The model under review builds one solid part; all positions refer to its coordinate system, in mm. Face numbers are marked on the shaded views. A direction names the side the tool comes from. Coordinates: 2 decimals unless noted, no trailing zeros. Write each loop counter-clockwise with the first axis right and the second up, starting at its lowest first coordinate (ties: lowest second). Pieces come first, ordered by that corner, then holes. Notation, with made-up numbers: (55.25, 69.5) - (106.25, 69.5) arc R33 cw to (106.25, 99.5) - close; hole circle Ø7 at (-31.5, 68). An arc over 180 degrees is marked (long way). Use one line per item in the form item = value. Start each with the question number.
```python
from build123d import *

# Parameters (mm, degrees)
F1_DEPTH = 7.874
F2_W     = 8.7442621589
F2_H     = 21.2777052075
F2_W_2   = 23.6095096916
F3_DEPTH = 6.35
F4_W     = 9.0357400477
F4_H     = 21.2777052075
F5_DEPTH = 17.272
F6_W     = 9.0357400477
F6_H     = 8.01557675
F7_DEPTH = 7.874
F8_W     = 3.937
F8_H     = 13.2621284574
F9_DEPTH = 14.986


with BuildPart() as f1:
    # F0 (on Front) → F1 (new body)
    with BuildSketch(Plane.XZ):
        Polygon((36.1429499462, 39.2034426332), (-43.4298366308, 39.2034426332), (-43.4298366308, 21.4234422892), (-21.2777052075, -14.1365574673), (13.9908185229, -14.1365574673), (36.1429499462, 21.4234422892), align=None)
    extrude(amount=F1_DEPTH)

    # F2 (on face) → F3 (join)
    with BuildSketch(Plane.XZ.offset(7.874)):
        with Locations((-20.6947550178, 28.5645900294)):
            Rectangle(F2_W, F2_H)
        with Locations((-4.5178690925, 28.5645900294)):
            Rectangle(F2_W_2, F2_H)
    extrude(amount=F3_DEPTH)

    # F4 (on face) → F5 (join)
    with BuildSketch(Plane.XZ.offset(14.224)):
        with Locations((-20.5490160733, 28.5645900294)):
            Rectangle(F4_W, F4_H)
    extrude(amount=F5_DEPTH)

    # F6 (on face) → F7 (cut)
    with BuildSketch(Plane.XZ.offset(31.496)):
        with Locations((-20.5490160733, 21.9335258007)):
            Rectangle(F6_W, F6_H)
    extrude(amount=-F7_DEPTH, mode=Mode.SUBTRACT)

    # F8 (on face) → F9 (join)
    with BuildSketch(Plane.YZ.offset(-16.0311460495)):
        with Locations((-29.5275, 32.5723784044)):
            Rectangle(F8_W, F8_H)
    extrude(amount=F9_DEPTH)


solid = f1.part
```
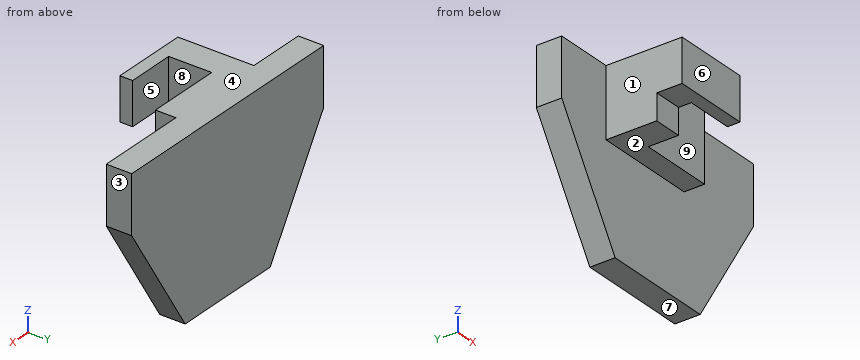
1. For the marked faces 1, 2, 3, 4 and 5, list the 3-axis set-ups (+Z, -Z, +X, -X, +Y, -Y) from which the entire face can be reached by the end or side of a thin tool; tool diameter is ignored.
2. For L1, parallel to Y at x = -14, z = 24.5; L2, parallel to Y at x = -33.5, z = 15; L3, parallel to Z at x = -24, y = -16.5, list the stretches that pass through material, from the lowest coordinate up.
3. Take a section at C-C (y = -4). State the section outline as (x, z) points, plus the area to 3 significant figures.
4. Take a section at D-D (x = 12). State the section outline as (y, z) points.
5. Take a section at A-A (x = -11). State the section outline as (y, z) points.
6. Take a section at B-B (z = 29.5). State the section outline as (x, y) points, plus the area to 3 significant figures.
7. For P1, Ø5, axis at y = -26.5, z = 26.5, coming from the +X side; P2, Ø3, axis at y = -11, z = 33.5, coming from the +X side; P3, Ø6, axis at x = -23.5, y = -13, coming from the -Z side; P4, Ø6.5, axis at x = -4, z = 25.5, coming from the -Y side, all flat-tipped, find the tip position at first contact; note any pin that passes through.
8. The part is to be moulded in two halves that separate along Y. For the marked faces 6, 7, 8 and 9, say which applies: released by +Y, released by -Y, zero draft, split by the parting line, or undercut.
Returned:
q1.face_1 = +Z, -Z, -X, -Y
q1.face_2 = -Z, +X, -X, -Y
q1.face_3 = +Z, -Z, +X, +Y, -Y
q1.face_4 = +Z, +X, -X, +Y, -Y
q1.face_5 = +Z, -Z, +X
q2.L1 = -14.22 to 0
q2.L2 = -7.87 to 0
q2.L3 = 17.93 to 39.2
q3.outline = (-43.43, 21.42) - (-21.28, -14.14) - (13.99, -14.14) - (36.14, 21.42) - (36.14, 39.2) - (-43.43, 39.2) - close
q3.area = 3,460 mm²
q4.outline = (-7.87, -14.14) - (0, -14.14) - (0, 39.2) - (-7.87, 39.2) - close
q5.outline = (-31.5, 25.94) - (-27.56, 25.94) - (-27.56, 39.2) - (-31.5, 39.2) - close; (-14.22, 17.93) - (-7.87, 17.93) - (-7.87, -14.14) - (0, -14.14) - (0, 39.2) - (-14.22, 39.2) - close
q6.outline = (-43.43, -7.87) - (-25.07, -7.87) - (-25.07, -31.5) - (-1.05, -31.5) - (-1.05, -27.56) - (-16.03, -27.56) - (-16.03, -14.22) - (7.29, -14.22) - (7.29, -7.87) - (36.14, -7.87) - (36.14, 0) - (-43.43, 0) - close
q6.area = 1,050 mm²
q7.P1 = -1.05
q7.P2 = 7.29
q7.P3 = 17.93
q7.P4 = -31.5
q8.face_6 = released by -Y
q8.face_7 = zero draft
q8.face_8 = undercut
q8.face_9 = undercut
